```python
from build123d import *

# Parameters (mm, degrees)
SKETCH_1_W          = 50
SKETCH_1_H          = 13
EXTRUDE_4_DEPTH     = 2
SKETCH_6_W          = 5
SKETCH_6_H          = 13
EXTRUDE_5_DEPTH     = 5
SKETCH_7_R          = 1.5
CUT_EXTRUDE_2_DEPTH = 5
SKETCH_8_W          = 5
SKETCH_8_H          = 13
EXTRUDE_6_DEPTH     = 5
SKETCH_9_W          = 3
SKETCH_9_H          = 9
CUT_EXTRUDE_3_DEPTH = 5
SKETCH_10_W         = 2
SKETCH_10_H         = 3
CUT_EXTRUDE_4_DEPTH = 5


with BuildPart() as part:
    # Эскиз1 → Бобышка-Вытянуть4 (new body)
    with BuildSketch(Plane.XY):
        Rectangle(SKETCH_1_W, SKETCH_1_H)
    extrude(amount=EXTRUDE_4_DEPTH)

    # Эскиз6 → Бобышка-Вытянуть5 (add)
    with BuildSketch(Plane.XY.offset(2)):
        with Locations((-22.5, 0)):
            Rectangle(SKETCH_6_W, SKETCH_6_H)
    extrude(amount=EXTRUDE_5_DEPTH)

    # Эскиз7 → Вырез-Вытянуть2 (cut)
    with BuildSketch(Plane(origin=(-20, 0, 0), x_dir=(0, 0, -1), z_dir=(1, 0, 0))):
        with Locations((-4.5, 0)):
            Circle(SKETCH_7_R)
    extrude(amount=-CUT_EXTRUDE_2_DEPTH, mode=Mode.SUBTRACT)

    # Эскиз8 → Бобышка-Вытянуть6 (add)
    with BuildSketch(Plane.XY.offset(2)):
        with Locations((22.5, 0)):
            Rectangle(SKETCH_8_W, SKETCH_8_H)
    extrude(amount=EXTRUDE_6_DEPTH)

    # Эскиз9 → Вырез-Вытянуть3 (cut)
    with BuildSketch(Plane.ZY.offset(-20)):
        with Locations((3.5, 0)):
            Rectangle(SKETCH_9_W, SKETCH_9_H)
    extrude(amount=-CUT_EXTRUDE_3_DEPTH, mode=Mode.SUBTRACT)

    # Эскиз10 → Вырез-Вытянуть4 (cut)
    with BuildSketch(Plane.ZY.offset(-20)):
        with Locations((6, 0)):
            Rectangle(SKETCH_10_W, SKETCH_10_H)
    extrude(amount=-CUT_EXTRUDE_4_DEPTH, mode=Mode.SUBTRACT)


solid = part.part
```
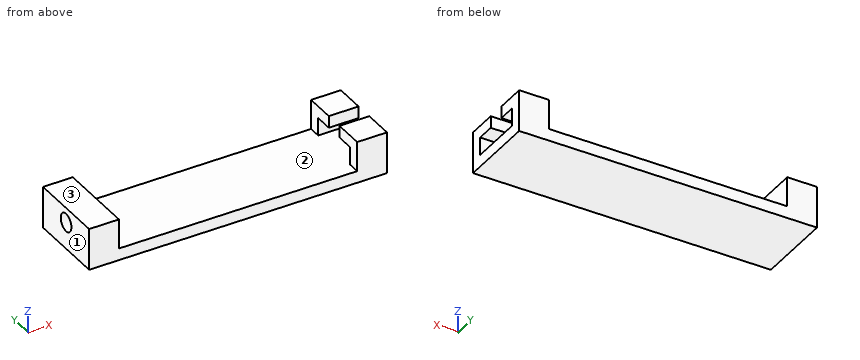
Verification items for the finished model (mm, model axes). Face numbers are marked on the shaded views. Coordinates: 2 decimals unless noted, no trailing zeros. Write each loop counter-clockwise with the first axis right and the second up, starting at its lowest first coordinate (ties: lowest second). Pieces come first, ordered by that corner, then holes. Notation, with made-up numbers: M -40,40.25 L -31,40.25 A11 ccw -31,49.25 Z; hole C 83.5,29.5 d10. An arc over 180 degrees is marked long. Answer as a JSON object with one key per item and string values. Group by question number.
(1) Material ranges on line 1 (Y direction, x = -22.8, z = 4.5); line 2 (X direction, y = -2, z = 6.25); line 3 (X direction, y = -3.75, z = 4), recorded low to high.
(2) Gauge pin test, flat ends, axial feed: pin 1 (2 mm diameter, centred on x = -7, y = 5, fed in from -Z); pin 2 (2 mm diameter, centred on x = -18.5, z = 6.5, fed in from +Y); pin 3 (6.5 mm diameter, centred on x = 1.5, y = -0.5, fed in from +Z). Record the tip position at first contact, or that the pin passes through.
(3) Cross-section at B-B, the plane z = 2.5. Record the cut outline in (x, y).
(4) Cross-section at A-A, the plane y = 3.5. Record the cut outline in (x, z), and give its area (3 significant figures).
(5) Cross-section at D-D, the plane y = 0. Record the cut outline in (x, z), and give its area (3 significant figures).
(6) Release check for a two-part mould opening along X. For the marked faces 1, 2 and 3 record: +X half, -X half, draft (parallel to the pull), parting line (faces both ways), or undercut.
(7) Cross-section at C-C, the plane z = 4.5. Record the cut outline in (x, y), and give its area (3 significant figures).
Reply:
{
 "1": {"line 1": "-6.5 to -1.5, 1.5 to 6.5", "line 2": "-25 to -20, 20 to 25", "line 3": "-25 to -20"},
 "2": {"pin 1": "z = 0", "pin 2": "through", "pin 3": "z = 2"},
 "3": {"outline": "M -25,-6.5 L -20,-6.5 L -20,6.5 L -25,6.5 Z; M 20,-6.5 L 25,-6.5 L 25,-4.5 L 20,-4.5 Z; M 20,4.5 L 25,4.5 L 25,6.5 L 20,6.5 Z"},
 "4": {"outline": "M -25,0 L 25,0 L 25,2 L -20,2 L -20,7 L -25,7 Z; M 20,5 L 25,5 L 25,7 L 20,7 Z", "area": "135 mm²"},
 "5": {"outline": "M -25,0 L 25,0 L 25,2 L -20,2 L -20,3 L -25,3 Z; M -25,6 L -20,6 L -20,7 L -25,7 Z", "area": "110 mm²"},
 "6": {"face 1": "-X half", "face 2": "undercut", "face 3": "draft"},
 "7": {"outline": "M -25,-6.5 L -20,-6.5 L -20,-1.5 L -25,-1.5 Z; M -25,1.5 L -20,1.5 L -20,6.5 L -25,6.5 Z; M 20,-6.5 L 25,-6.5 L 25,-4.5 L 20,-4.5 Z; M 20,4.5 L 25,4.5 L 25,6.5 L 20,6.5 Z", "area": "70.0 mm²"}
}
